For this review, take the finished solid that the model builds, in its own axes (mm). A direction names the side the tool comes from. Round coordinates to 2 decimals unless told otherwise and drop trailing zeros. Loops run counter-clockwise (first coordinate to the right, second up) from the corner with the lowest first, then second, coordinate; pieces in that order, holes last. Notation, with made-up numbers: (28, 3) -> (50, 3) arc R31 ccw to (50, 41) -> close; hole circle Ø10 at (54, -27.75). An arc over 180 degrees is marked (long way). One line per question, with ' | ' between items. Start each with the question number.
1. Consider section C-C (x = 87). Write out the cut boundary in (y, z).
2. Consider section B-B (z = 33.5). Write out the cut boundary in (x, y).
3. Consider section A-A (y = 34.5). Write out the cut boundary in (x, z).
4. Wall thickness on line 1 along Y through (x, z) = (-25.5, 24.5); line 2 along Y through (x, z) = (73, 17); line 3 along Y through (x, z) = (45.5, 47.5): over which ranges is each line inside the solid? List them lowest first.
5. Consider section D-D (z = 14.5). Write out the cut boundary in (x, y).
6. Draft analysis for pull direction Z (two halves, no side actions). For faces 4 (the face through (29, 40, 31)), 5 (the face through (-15, 32, 40)), 6 (the face through (33, -35, 10)), 7 (the face through (56, 1, 0)), state which applies: pulls with the +Z half, pulls with the -Z half, needs draft (parallel to the pull), parting line crosses it, or undercut.
7. For faces 1 (the face through (98, -10, 36)), 2 (the face through (29.28, 30.14, 39.51)), 3 (the face through (29, 35, 20)), list the 3-axis set-ups (+Z, -Z, +X, -X, +Y, -Y) from which the entire face can be reached by the end or side of a thin tool; tool diameter is ignored.
8. For pin 1 Ø6 at (x, y) = (51.5, -32) entering from +Z; pin 2 Ø7.5 at (x, z) = (53, 42) entering from +Y; pin 3 Ø4.5 at (x, y) = (-12.5, -28.5) entering from +Z, all flat-tipped, find the tip position at first contact; note any pin that passes through.
```python
from build123d import *

# Parameters (mm, degrees)
F1_DEPTH = 50
F2_W     = 40
F2_H     = 10
F3_DEPTH = 30
F4_DEPTH = 10
F5_DEPTH = 20


# Not quite as in the source:
# - a pattern or mirror of a feature is missing from the dataset's text; its kind, count and spacing are read off the source's solid


with BuildPart() as f1:
    # F0 (on Top) → F1 (new body)
    with BuildSketch(Plane.XY):
        with BuildLine():
            Line((-35, -25), (-35, -40))
            Line((-35, -40), (115, -40))
            Line((115, -40), (115, 40))
            Line((115, 40), (-35, 40))
            Line((-35, 40), (-35, 25))
            Line((-35, 25), (0, 25))
            ThreePointArc((0, 25), (25, 0), (0, -25))
            Line((0, -25), (-35, -25))
        make_face()
    extrude(amount=F1_DEPTH)

    # F2 (on face) → F3 (cut)
    with BuildSketch(Plane.XZ.offset(40)):
        with Locations((-15, 45)):
            Rectangle(F2_W, F2_H)
        Polygon((115, 50), (55, 50), (73, 35), (91, 20), (103, 10), (115, 0), align=None)
    f3 = extrude(amount=-F3_DEPTH, mode=Mode.SUBTRACT)

    # F3_copies: F3 across plane
    add(f3.mirror(Plane.ZX), mode=Mode.SUBTRACT)

    # F2 (on face) → F4 (cut)
    with BuildSketch(Plane.XZ.offset(40)):
        Polygon((91, 20), (-35, 20), (-35, 10), (103, 10), align=None)
    f4 = extrude(amount=-F4_DEPTH, mode=Mode.SUBTRACT)

    # F4_copies: F4 across plane
    add(f4.mirror(Plane.ZX), mode=Mode.SUBTRACT)

    # F2 (on face) → F5 (cut)
    with BuildSketch(Plane.XZ.offset(40)):
        with BuildLine():
            Line((55, 50), (25, 50))
            ThreePointArc((25, 50), (29.3933982822, 39.3933982822), (40, 35))
            Line((40, 35), (73, 35))
            Line((73, 35), (55, 50))
        make_face()
    f5 = extrude(amount=-F5_DEPTH, mode=Mode.SUBTRACT)

    # F5_copies: F5 across plane
    add(f5.mirror(Plane.ZX), mode=Mode.SUBTRACT)


solid = f1.part
```
Answer block:
1) outline: (-40, 0) -> (40, 0) -> (40, 10) -> (30, 10) -> (30, 20) -> (40, 20) -> (40, 23.33) -> (10, 23.33) -> (10, 50) -> (-10, 50) -> (-10, 23.33) -> (-40, 23.33) -> (-40, 20) -> (-30, 20) -> (-30, 10) -> (-40, 10) -> close
2) outline: (-35, -40) -> (74.8, -40) -> (74.8, -10) -> (115, -10) -> (115, 10) -> (74.8, 10) -> (74.8, 40) -> (-35, 40) -> (-35, 25) -> (0, 25) arc R25 cw to (0, -25) -> (-35, -25) -> close
3) outline: (-35, 0) -> (115, 0) -> (103, 10) -> (-35, 10) -> close; (-35, 20) -> (91, 20) -> (73, 35) -> (40, 35) arc R15 cw to (25, 50) -> (5, 50) -> (5, 40) -> (-35, 40) -> close
4) line 1: y = -40 to -25, 25 to 40 | line 2: y = -30 to 30 | line 3: y = -20 to 20
5) outline: (-35, -30) -> (97.6, -30) -> (97.6, -10) -> (115, -10) -> (115, 10) -> (97.6, 10) -> (97.6, 30) -> (-35, 30) -> (-35, 25) -> (0, 25) arc R25 cw to (0, -25) -> (-35, -25) -> close
6) face 4: needs draft | face 5: pulls with the +Z half | face 6: undercut | face 7: pulls with the -Z half
7) face 1: +Z, +X, -Y | face 2: +Z, +X, +Y | face 3: +X, -X, +Y
8) pin 1: stops at z = 35 | pin 2: stops at y = 20 | pin 3: stops at z = 40
